Here's how the part is built. I have some questions about the finished solid (model axes, mm). Face numbers are marked on the shaded views. Give positions to 0.01 mm unless a question says otherwise; leave off trailing zeros. Order: outer loops, then holes, each group sorted by start corner. A loop starts at its lowest first (then second) coordinate and runs counter-clockwise, first axis right, second up. Notation, with made-up numbers: M -9,34.25 L 13,34.25 A26 cw 13,52.25 Z; hole C 87.5,-18 d8. An arc over 180 degrees is marked long. Use one line per item in the form item = value.
from build123d import *

# Parameters (mm, degrees)
SKETCH1_R           = 7.75
EXTRUDE1_DEPTH      = 17
EXTRUDE2_DEPTH      = 3.7
EXTRUDE2_DEPTH_BACK = 3.7
SKETCH3_R           = 8.5
EXTRUDE3_DEPTH      = 4
EXTRUDE3_DEPTH_BACK = 4
SKETCH4_R           = 5
SKETCH4_R_2         = 1.53125
EXTRUDE4_DEPTH      = 8.7500001
EXTRUDE4_DEPTH_BACK = 8.7500001
SKETCH5_R           = 5.8
EXTRUDE5_DEPTH      = 6.1
EXTRUDE5_DEPTH_BACK = 6.1


with BuildPart() as part:
    # Sketch1 → Extrude1 (new body)
    with BuildSketch(Plane.XY):
        Circle(SKETCH1_R)
    extrude(amount=EXTRUDE1_DEPTH)

    # Sketch2 → Extrude2 (cut, two sides)
    with BuildSketch(Plane(origin=(0, 0, 0), x_dir=(0, 0, -1), z_dir=(1, 0, 0))) as extrude2_sk:
        with BuildLine():
            Line((-17, 7.75), (-17, -7.81981982))
            Line((-17, -7.81981982), (-8.981869421, -7.81981982))
            ThreePointArc((-8.981869421, -7.81981982), (-5.800105265, -0.048558495), (-8.914364589, 7.75))
            Line((-8.914364589, 7.75), (-17, 7.75))
        make_face()
    extrude(amount=EXTRUDE2_DEPTH, mode=Mode.SUBTRACT)
    extrude(extrude2_sk.sketch, amount=-EXTRUDE2_DEPTH_BACK, mode=Mode.SUBTRACT)

    # Sketch3 → Extrude3 (cut, two sides)
    with BuildSketch(Plane(origin=(0, 0, 0), x_dir=(0, 0, -1), z_dir=(1, 0, 0))) as extrude3_sk:
        with Locations((-17, 0)):
            Circle(SKETCH3_R)
    extrude(amount=EXTRUDE3_DEPTH, mode=Mode.SUBTRACT)
    extrude(extrude3_sk.sketch, amount=-EXTRUDE3_DEPTH_BACK, mode=Mode.SUBTRACT)

    # Sketch4 → Extrude4 (cut, two sides)
    with BuildSketch(Plane(origin=(0, 0, 0), x_dir=(0, 0, -1), z_dir=(1, 0, 0))) as extrude4_sk:
        with Locations((-17, 0)):
            Circle(SKETCH4_R)
        with Locations((-3.0625, 0)):
            Circle(SKETCH4_R_2)
    extrude(amount=EXTRUDE4_DEPTH, mode=Mode.SUBTRACT)
    extrude(extrude4_sk.sketch, amount=-EXTRUDE4_DEPTH_BACK, mode=Mode.SUBTRACT)

    # Sketch5 → Extrude5 (cut, two sides)
    with BuildSketch(Plane(origin=(0, 0, 0), x_dir=(0, 0, -1), z_dir=(1, 0, 0))) as extrude5_sk:
        with Locations((-16.84375, 0)):
            Circle(SKETCH5_R)
    extrude(amount=EXTRUDE5_DEPTH, mode=Mode.SUBTRACT)
    extrude(extrude5_sk.sketch, amount=-EXTRUDE5_DEPTH_BACK, mode=Mode.SUBTRACT)


solid = part.part
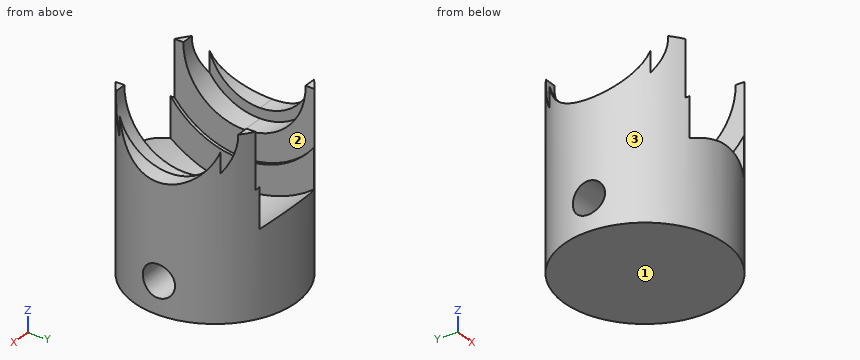
Q1. I want a section at B-B on z = 14.5. Write out the boundary of the cut face in (x, y), then the cut area to 3 significant figures.
Found:
outline = M -6.43,-4.33 A7.75 ccw -6.1,-4.78 L -6.1,-4.33 Z; M -6.43,4.33 L -6.1,4.33 L -6.1,4.78 A7.75 ccw Z; M -5.65,-5.31 A7.75 ccw -4,-6.64 L -4,-5.31 Z; M -5.65,5.31 L -4,5.31 L -4,6.64 A7.75 ccw Z; M 4,-6.64 A7.75 ccw 5.65,-5.31 L 4,-5.31 Z; M 4,5.31 L 5.65,5.31 A7.75 ccw 4,6.64 Z; M 6.1,-4.78 A7.75 ccw 6.43,-4.33 L 6.1,-4.33 Z; M 6.1,4.33 L 6.43,4.33 A7.75 ccw 6.1,4.78 Z
area = 5.11 mm²
Q2. I'm going to push flat-ended pins straight in: pin 1 Ø8 at (x, y) = (2, 4) entering from -Z; pin 2 Ø4 at (y, z) = (-5.5, 3) entering from -X; pin 3 Ø1 at (y, z) = (-1.5, 2.5) entering from -X; pin 4 Ø5 at (x, z) = (-4, 12) entering from -Y. Where does each tip first touch, or does it pass through?
Found:
pin_1 = 0
pin_2 = -6.91
pin_3 = -7.66
pin_4 = -6.81
Q3. I want a section at C-C on z = 7.5. Write out the boundary of the cut face in (x, y).
Found:
outline = C 0,0 d15.5; hole M -3.7,-5.93 L 3.7,-5.93 L 3.7,5.93 L -3.7,5.93 Z
Q4. I want a section at D-D on y = 4. Write out the boundary of the cut face in (x, z).
Found:
outline = M -6.64,0 L 6.64,0 L 6.64,14 L 6.1,14 L 6.1,12.64 L 4,12.64 L 4,9.5 L 3.7,9.5 L 3.7,6.54 L -3.7,6.54 L -3.7,9.5 L -4,9.5 L -4,12.64 L -6.1,12.64 L -6.1,14 L -6.64,14 Z
Q5. I need wall thicknesses on L1, parallel to Z at x = 2.75, y = 0; L2, parallel to Z at x = 6, y = 0; L3, parallel to Y at x = 4, z = 1. Which ranges of each line are inside material? Lowest first, please.
Found:
L1 = 0 to 1.53, 4.59 to 5.8
L2 = 0 to 1.53, 4.59 to 11.04
L3 = -6.64 to 6.64
Q6. Thinking about a two-plate mould opening in Y: for the marked faces 1, 2 and 3, which applies, +Y half, -Y half, draft (parallel to the pull), parting line (faces both ways), or undercut?
Found:
face_1 = draft
face_2 = undercut
face_3 = parting line
